Can you work these out from the model? Positions are in its coordinate system, mm. A direction names the side the tool comes from. Round coordinates to 2 decimals unless told otherwise and drop trailing zeros. Write each loop counter-clockwise with the first axis right and the second up, starting at its lowest first coordinate (ties: lowest second). Pieces come first, ordered by that corner, then holes.
Q1. Please list where these lines run through material, in increasing order: line 1 along X through (y, z) = (1.85, 5); line 2 along X through (y, z) = (1.3, -5.25); line 3 along Z through (x, y) = (1, 2.7).
Q2. I'm going to push flat-ended pins straight in: pin 1 Ø3 at (x, z) = (0, 0) entering from +Y; pin 2 Ø1 at (y, z) = (2.5, -2.5) entering from +X; pin 3 Ø6 at (x, z) = (5, -4) entering from -Y. Where does each tip first touch, or does it pass through?
Q3. If we section it at C-C (z = -2.25): Please give me the cut outline in (x, y).
Q4. We'd pull the mould along X, two halves only. Please class faces 1 (the flat face through (1.22, 1.48, -6.78)), 2 (the flat face through (0.17, 1.48, -6.19)), 3 (the flat face through (0, 3, -2)), 4 (the flat face through (-4.45, 1.48, 5.26)): +X half, -X half, draft (parallel to the pull), parting line (faces both ways), or undercut.
Q5. For faces 5 (the cylindrical face through (3.213, 1.479, 4.464)), 6 (the flat face through (-0.17, 1.48, 6.19)), 7 (the flat face through (-6.024, 1.479, 1.264)), 8 (the flat face through (3.239, 1.479, -5.274)), 9 (the flat face through (5.274, 1.479, 3.239)), which set-ups out of +Z, -Z, +X, -X, +Y, -Y let a thin tool reach every point of the face, with its end or its side?
Q6. If we section it at A-A (x = 0.75): Please give me the cut outline in (y, z).
Q7. If we section it at B-B (z = 1.25): Please give me the cut outline in (x, y).
from build123d import *

# Parameters (mm, degrees)
SKETCH1_R               = 7
BOSS_EXTRUDE1_DEPTH     = 3
CUT_EXTRUDE1_DEPTH      = 11.344080433
CUT_EXTRUDE1_DEPTH_BACK = 3
SKETCH5_R               = 1.6
CUT_EXTRUDE2_DEPTH      = 3


with BuildPart() as part:
    # Sketch1 → Boss-Extrude1 (new body)
    with BuildSketch(Plane(origin=(0, 0, 0), x_dir=(1, 0, 0), z_dir=(0, 1, 0))):
        with Locations(Location((0, 0, 0), (0, 0, 270))):
            Circle(SKETCH1_R)
    extrude(amount=BOSS_EXTRUDE1_DEPTH)

    # Sketch2 → Cut-Extrude1 (cut, two sides: drawn at the far end of the back side and taken through both)
    with BuildSketch(Plane(origin=(0, 3, 0), x_dir=(1, 0, 0), z_dir=(0, 1, 0)).offset(-CUT_EXTRUDE1_DEPTH_BACK)):
        with BuildLine():
            ThreePointArc((-1.079936716, 5.392933959), (-0.542615529, 5.473168039), (0, 5.5))
            Line((0, 5.5), (0, 7))
            ThreePointArc((0, 7), (-7, 0), (0, -7))
            Line((0, -7), (0, -5.5))
            Line((0, -5.5), (-0.341646298, -6.893330445))
            ThreePointArc((-0.341646298, -6.893330445), (-0.386932449, -6.955031571), (-0.462583878, -6.966638711))
            Line((-0.462583878, -6.966638711), (-1.996653446, -6.590483011))
            ThreePointArc((-1.996653446, -6.590483011), (-2.058354572, -6.54519686), (-2.069961712, -6.469545431))
            Line((-2.069961712, -6.469545431), (-1.761214349, -5.210386168))
            ThreePointArc((-1.761214349, -5.210386168), (-2.266665187, -5.011210326), (-2.75, -4.763139721))
            Line((-2.75, -4.763139721), (-3.742539596, -5.798976134))
            ThreePointArc((-3.742539596, -5.798976134), (-3.812609116, -5.8297678), (-3.883928745, -5.801994164))
            Line((-3.883928745, -5.801994164), (-5.024394113, -4.709198988))
            ThreePointArc((-5.024394113, -4.709198988), (-5.055185779, -4.639129468), (-5.027412143, -4.567809838))
            Line((-5.027412143, -4.567809838), (-4.130449452, -3.63171961))
            ThreePointArc((-4.130449452, -3.63171961), (-4.468594797, -3.206502852), (-4.763139721, -2.75))
            Line((-4.763139721, -2.75), (-6.140622431, -3.15079085))
            ThreePointArc((-6.140622431, -3.15079085), (-6.216700249, -3.142422455), (-6.264578041, -3.082709966))
            Line((-6.264578041, -3.082709966), (-6.705852434, -1.566088898))
            ThreePointArc((-6.705852434, -1.566088898), (-6.69748404, -1.490011081), (-6.63777155, -1.442133288))
            Line((-6.63777155, -1.442133288), (-5.392933959, -1.079936716))
            ThreePointArc((-5.392933959, -1.079936716), (-5.473168039, -0.542615529), (-5.5, 0))
            Line((-5.5, 0), (-6.893330445, 0.341646298))
            ThreePointArc((-6.893330445, 0.341646298), (-6.955031571, 0.386932449), (-6.966638711, 0.462583878))
            Line((-6.966638711, 0.462583878), (-6.590483011, 1.996653446))
            ThreePointArc((-6.590483011, 1.996653446), (-6.54519686, 2.058354572), (-6.469545431, 2.069961712))
            Line((-6.469545431, 2.069961712), (-5.210386168, 1.761214349))
            ThreePointArc((-5.210386168, 1.761214349), (-5.011210326, 2.266665187), (-4.763139721, 2.75))
            Line((-4.763139721, 2.75), (-5.798976134, 3.742539596))
            ThreePointArc((-5.798976134, 3.742539596), (-5.8297678, 3.812609116), (-5.801994164, 3.883928745))
            Line((-5.801994164, 3.883928745), (-4.709198988, 5.024394113))
            ThreePointArc((-4.709198988, 5.024394113), (-4.639129468, 5.055185779), (-4.567809838, 5.027412143))
            Line((-4.567809838, 5.027412143), (-3.63171961, 4.130449452))
            ThreePointArc((-3.63171961, 4.130449452), (-3.206502852, 4.468594797), (-2.75, 4.763139721))
            Line((-2.75, 4.763139721), (-3.15079085, 6.140622431))
            ThreePointArc((-3.15079085, 6.140622431), (-3.142422455, 6.216700249), (-3.082709966, 6.264578041))
            Line((-3.082709966, 6.264578041), (-1.566088898, 6.705852434))
            ThreePointArc((-1.566088898, 6.705852434), (-1.490011081, 6.69748404), (-1.442133288, 6.63777155))
            Line((-1.442133288, 6.63777155), (-1.079936716, 5.392933959))
        make_face()
        with BuildLine():
            Line((0, 7), (0, 5.5))
            Line((0, 5.5), (0.341646298, 6.893330445))
            ThreePointArc((0.341646298, 6.893330445), (0.386932449, 6.955031571), (0.462583878, 6.966638711))
            Line((0.462583878, 6.966638711), (1.996653446, 6.590483011))
            ThreePointArc((1.996653446, 6.590483011), (2.058354572, 6.54519686), (2.069961712, 6.469545431))
            Line((2.069961712, 6.469545431), (1.761214349, 5.210386168))
            ThreePointArc((1.761214349, 5.210386168), (2.266665187, 5.011210326), (2.75, 4.763139721))
            Line((2.75, 4.763139721), (3.742539596, 5.798976134))
            ThreePointArc((3.742539596, 5.798976134), (3.812609116, 5.8297678), (3.883928745, 5.801994164))
            Line((3.883928745, 5.801994164), (5.024394113, 4.709198988))
            ThreePointArc((5.024394113, 4.709198988), (5.055185779, 4.639129468), (5.027412143, 4.567809838))
            Line((5.027412143, 4.567809838), (4.130449452, 3.63171961))
            ThreePointArc((4.130449452, 3.63171961), (4.468594797, 3.206502852), (4.763139721, 2.75))
            Line((4.763139721, 2.75), (6.140622431, 3.15079085))
            ThreePointArc((6.140622431, 3.15079085), (6.216700249, 3.142422455), (6.264578041, 3.082709966))
            Line((6.264578041, 3.082709966), (6.705852434, 1.566088898))
            ThreePointArc((6.705852434, 1.566088898), (6.69748404, 1.490011081), (6.63777155, 1.442133288))
            Line((6.63777155, 1.442133288), (5.392933959, 1.079936716))
            ThreePointArc((5.392933959, 1.079936716), (5.473168039, 0.542615529), (5.5, 0))
            Line((5.5, 0), (6.893330445, -0.341646298))
            ThreePointArc((6.893330445, -0.341646298), (6.955031571, -0.386932449), (6.966638711, -0.462583878))
            Line((6.966638711, -0.462583878), (6.590483011, -1.996653446))
            ThreePointArc((6.590483011, -1.996653446), (6.54519686, -2.058354572), (6.469545431, -2.069961712))
            Line((6.469545431, -2.069961712), (5.210386168, -1.761214349))
            ThreePointArc((5.210386168, -1.761214349), (5.011210326, -2.266665187), (4.763139721, -2.75))
            Line((4.763139721, -2.75), (5.798976134, -3.742539596))
            ThreePointArc((5.798976134, -3.742539596), (5.8297678, -3.812609116), (5.801994164, -3.883928745))
            Line((5.801994164, -3.883928745), (4.709198988, -5.024394113))
            ThreePointArc((4.709198988, -5.024394113), (4.639129468, -5.055185779), (4.567809838, -5.027412143))
            Line((4.567809838, -5.027412143), (3.63171961, -4.130449452))
            ThreePointArc((3.63171961, -4.130449452), (3.206502852, -4.468594797), (2.75, -4.763139721))
            Line((2.75, -4.763139721), (3.15079085, -6.140622431))
            ThreePointArc((3.15079085, -6.140622431), (3.142422455, -6.216700249), (3.082709966, -6.264578041))
            Line((3.082709966, -6.264578041), (1.566088898, -6.705852434))
            ThreePointArc((1.566088898, -6.705852434), (1.490011081, -6.69748404), (1.442133288, -6.63777155))
            Line((1.442133288, -6.63777155), (1.079936716, -5.392933959))
            ThreePointArc((1.079936716, -5.392933959), (0.542615529, -5.473168039), (0, -5.5))
            Line((0, -5.5), (0, -7))
            ThreePointArc((0, -7), (4.949747468, -4.949747468), (7, 0))
            ThreePointArc((7, 0), (4.949747468, 4.949747468), (0, 7))
        make_face()
    extrude(amount=CUT_EXTRUDE1_DEPTH + CUT_EXTRUDE1_DEPTH_BACK, mode=Mode.SUBTRACT)

    # Sketch5 → Cut-Extrude2 (cut)
    with BuildSketch(Plane(origin=(0, 3, 0), x_dir=(1, 0, 0), z_dir=(0, 1, 0))):
        with Locations(Location((0, 0, 0), (0, 0, 270))):
            Circle(SKETCH5_R)
    extrude(amount=-CUT_EXTRUDE2_DEPTH, mode=Mode.SUBTRACT)


solid = part.part
A:
1. line 1: x = -4.72 to -2.98, -2.29 to 2.82, 4.54 to 4.73
1. line 2: x = -2.89 to 1.77, 3.22 to 4.46
1. line 3: z = -6.83 to -1.25, 1.25 to 5.41
2. pin 1: passes through
2. pin 2: stops at x = 6.58
2. pin 3: stops at y = 0
3. outline: (-5.02, 0) - (6.51, 0) - (6.51, 3) - (-5.02, 3) - close
4. face 1: +X half
4. face 2: undercut
4. face 3: draft
4. face 4: -X half
5. face 5: +Y, -Y
5. face 6: +Z, +Y, -Y
5. face 7: -X, +Y, -Y
5. face 8: -Z, +Y, -Y
5. face 9: +X, +Y, -Y
6. outline: (0, -6.9) - (3, -6.9) - (3, -1.41) - (0, -1.41) - close; (0, 1.41) - (3, 1.41) - (3, 5.45) - (0, 5.45) - close
7. outline: (-5.98, 0) - (-1, 0) - (-1, 3) - (-5.98, 3) - close; (1, 0) - (6.77, 0) - (6.77, 3) - (1, 3) - close
